from build123d import *

# Parameters (mm, degrees)
SKETCH_R     = 60
SKETCH_R_2   = 2.6
SKETCH_R_3   = 2.1
PAD_DEPTH    = 6
CHAMFER_SIZE = 2
POCKET_DEPTH = 3.2


with BuildPart() as part:
    # Sketch → Pad (new body)
    with BuildSketch(Plane.XZ):
        Circle(SKETCH_R)
        with Locations((-45, 0)):
            Circle(SKETCH_R_2, mode=Mode.SUBTRACT)
        with Locations((45, 0)):
            Circle(SKETCH_R_2, mode=Mode.SUBTRACT)
        with Locations((-30, 0)):
            Circle(SKETCH_R_3, mode=Mode.SUBTRACT)
        with Locations((30, 0)):
            Circle(SKETCH_R_3, mode=Mode.SUBTRACT)
        with Locations((0, 30)):
            Circle(SKETCH_R_3, mode=Mode.SUBTRACT)
        with Locations((0, -30)):
            Circle(SKETCH_R_3, mode=Mode.SUBTRACT)
    extrude(amount=PAD_DEPTH)

    # Chamfer
    chamfer_edges = [part.edges().sort_by_distance(p)[0] for p in [
        (-47.6, -6, 0),
        (42.4, -6, 0),
    ]]
    chamfer(chamfer_edges, length=CHAMFER_SIZE)

    # Sketch001 → Pocket (cut)
    with BuildSketch(Plane.XZ):
        Polygon((2, 33.464102), (-2, 33.464102), (-4, 30), (-2, 26.535898), (2, 26.535898), (4, 30), align=None)
        Polygon((32, 3.464102), (28, 3.464102), (26, 0), (28, -3.464102), (32, -3.464102), (34, 0), align=None)
        Polygon((2, -26.535898), (-2, -26.535898), (-4, -30), (-2, -33.464102), (2, -33.464102), (4, -30), align=None)
        Polygon((-32, 3.464102), (-34, 0), (-32, -3.464102), (-28, -3.464102), (-26, 0), (-28, 3.464102), align=None)
    extrude(amount=POCKET_DEPTH, mode=Mode.SUBTRACT)


solid = part.part
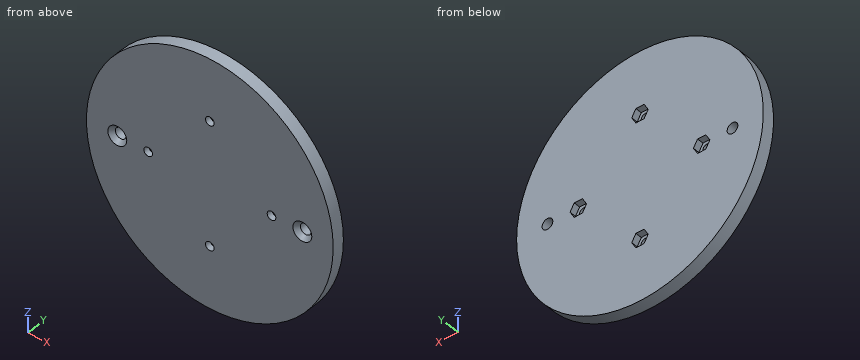
Build history of the part. All positions in model axes, mm. Round coordinates to 2 decimals unless told otherwise and drop trailing zeros. Write each loop counter-clockwise with the first axis right and the second up, starting at its lowest first coordinate (ties: lowest second). Pieces come first, ordered by that corner, then holes. Notation, with made-up numbers: M -26.75,-11 L -14.75,-11 A21 ccw -14.75,10 Z; hole C 67.5,48 d6. An arc over 180 degrees is marked long. Answer in a Markdown table with one row per item.
1. Saw through at D-D (z = -18). List the corners of the cut face in (x, y), and give its area (3 significant figures).
Geometry check:
| item | result |
|---|---|
| outline | M -57.24,-6 L 57.24,-6 L 57.24,0 L -57.24,0 Z |
| area | 687 mm2 |
2. Saw through at B-B (y = -2.3). List the corners of the cut face in (x, z), and give its area (3 significant figures).
Geometry check:
| item | result |
|---|---|
| outline | C 0,0 d120; hole C -45,0 d5.2; hole M -34,0 L -32,-3.46 L -28,-3.46 L -26,0 L -28,3.46 L -32,3.46 Z; hole M -4,-30 L -2,-33.46 L 2,-33.46 L 4,-30 L 2,-26.54 L -2,-26.54 Z; hole M -4,30 L -2,26.54 L 2,26.54 L 4,30 L 2,33.46 L -2,33.46 Z; hole M 26,0 L 28,-3.46 L 32,-3.46 L 34,0 L 32,3.46 L 28,3.46 Z; hole C 45,0 d5.2 |
| area | 11,100 mm2 |
3. Saw through at A-A (x = 0). List the corners of the cut face in (y, z), and give its area (3 significant figures).
Geometry check:
| item | result |
|---|---|
| outline | M -6,-60 L 0,-60 L 0,-33.46 L -3.2,-33.46 L -3.2,-32.1 L -6,-32.1 Z; M -6,-27.9 L -3.2,-27.9 L -3.2,-26.54 L 0,-26.54 L 0,26.54 L -3.2,26.54 L -3.2,27.9 L -6,27.9 Z; M -6,32.1 L -3.2,32.1 L -3.2,33.46 L 0,33.46 L 0,60 L -6,60 Z |
| area | 652 mm2 |
4. Saw through at C-C (x = 29.5). List the corners of the cut face in (y, z), and give its area (3 significant figures).
Geometry check:
| item | result |
|---|---|
| outline | M -6,-52.25 L 0,-52.25 L 0,-3.46 L -3.2,-3.46 L -3.2,-2.04 L -6,-2.04 Z; M -6,2.04 L -3.2,2.04 L -3.2,3.46 L 0,3.46 L 0,52.25 L -6,52.25 Z |
| area | 593 mm2 |
5. Flat gauge pins, fed straight in: P1, Ø1, axis at x = -0.5, y = -2.5, coming from the +Z side; P2, Ø3.5, axis at x = 0, z = -31, coming from the +Y side; P3, Ø3.5, axis at x = 0, y = -2, coming from the -Z side. Where does each tip first touch, or does it go through?
Geometry check:
| item | result |
|---|---|
| P1 | z = 60 |
| P2 | y = -3.2 |
| P3 | z = -60 |
6. Probe L1, parallel to Z at x = 0, y = -3.95; L2, parallel to Z at x = -46.5, y = -2.25; L3, parallel to Z at x = 29, y = -2.75. List the from-to ranges inside material, lowest first. Write a range as [from, to].
Geometry check:
| item | result |
|---|---|
| L1 | [-60, -32.1], [-27.9, 27.9], [32.1, 60] |
| L2 | [-37.92, -2.12], [2.12, 37.92] |
| L3 | [-52.53, -3.46], [3.46, 52.53] |
